Build history of the part. All positions in model axes, mm. A direction names the side the tool comes from. Round coordinates to 2 decimals unless told otherwise and drop trailing zeros. Loops run counter-clockwise (first coordinate to the right, second up) from the corner with the lowest first, then second, coordinate; pieces in that order, holes last. Notation, with made-up numbers: (31, 58.25) - (72, 58.25) arc R24 cw to (72, 73.25) - close; hole circle Ø11 at (-33.5, 32). An arc over 180 degrees is marked (long way). Use a Markdown table: item, result.
Autodesk Inventor part; units mm, degrees
ref_plane "РабПлоскость1" through (0, 0, 3) normal (0, 0, 1) x (1, 0, 0)
ref_plane "YZ Plane" through (0, 0, 0) normal (1, 0, 0) x (0, 1, 0)
ref_plane "XZ Plane" through (0, 0, 0) normal (0, 1, 0) x (-1, 0, 0)
ref_plane "РабПлоскость1" through (0, 0, 3) normal (0, 0, 1) x (1, 0, 0)
sketch "Эскиз1" plane through (0, 0, 3) normal (0, 0, 1) x (1, 0, 0)
  circle A0 centre (0, 0) radius 135
  circle A1 centre (0, 0) radius 101 construction
  line L0 (0, 0) -> (0, 184.3698) construction
  circle A2 centre (-37.8353, 93.6456) radius 27
  circle A3 centre (-92.2681, 41.0804) radius 27
  circle A4 centre (37.8353, 93.6456) radius 27
  circle A5 centre (92.2681, 41.0804) radius 27
  line L1 (0, 0) -> (37.8353, 93.6456) construction
  line L2 (0, 0) -> (92.2681, 41.0804) construction
  circle A6 centre (0, 0) radius 67
  line L3 (-135, 0) -> (135, 0)
  circle A7 centre (120, 0) radius 1.6 construction
  circle A8 centre (-120, 0) radius 1.6 construction
  circle A9 centre (120, 0) radius 8 construction
  circle A10 centre (-120, 0) radius 8 construction
  circle A11 centre (0, 120) radius 1.6 construction
  circle A12 centre (0, 120) radius 8 construction
  line L4 (0, 0) -> (-116.9134, -67.5) construction
  line L5 (0, 0) -> (116.9134, -67.5) construction
  point P0 (67, 0)
  point P1 (-67, 0)
  point P2 (-128, 0)
  point P3 (-112, 0)
  point P4 (112, 0)
  point P5 (128, 0)
  dimension "d0" = 54
  dimension "d3" = 202
  dimension "d4" = 34
  dimension "d5" = 34
  dimension "d9" = 16
  dimension "d11" = 120
  dimension "d12" = 22
  dimension "d13" = 44
extrude "Выдавливание1" add sketch "Эскиз1" along normal blind 6 contours L3 A6 A0 picked at (99.1742, 4.7591)
fillet "Сопряжение1" radius 5 4 edges at (-67, 0, 6) (-135, 0, 6) (67, 0, 6) (135, 0, 6)
equation "\"d5\" = d4"
equation "\"d13\" = 2 * d12"
properties part number "Фиксатор" material "По умолчанию1"
Q1. Drop flat-ended pins along their axis: pin 1 (2 mm diameter, centred on x = 14.5, z = 5, fed in from +Y); pin 2 (2 mm diameter, centred on x = 74.5, z = 6.5, fed in from +Y). Give the stop position or say it passes through.
Results found:
| item | result |
|---|---|
| pin 1 | stops at y = 134.32 |
| pin 2 | stops at y = 113.24 |
Q2. Cut at B-B, the plane x = -56.5. List the corners of the cut face in (y, z).
Results found:
| item | result |
|---|---|
| outline | (36.01, 3) - (74.14, 3) - (74.14, 9) - (36.01, 9) - close; (113.16, 3) - (122.61, 3) - (122.61, 9) - (113.16, 9) - close |
Q3. Which spindle directions (+Z, -Z, +X, -X, +Y, -Y) get a long thin tool onto all of the face, cutting with end or side? Do faces 4 (the face through (-68.45, 1.31, 6.04)), 5 (the face through (-66.515, 32.97, 5.958)). Say none if no direction does.
Results found:
| item | result |
|---|---|
| face 4 | +Z, -Z, -Y |
| face 5 | +Z, -Z |
Q4. Cut at C-C, the plane y = 117. List the corners of the cut face in (x, z).
Results found:
| item | result |
|---|---|
| outline | (-67.35, 3) - (-51.38, 3) - (-51.38, 9) - (-67.35, 9) - close; (-24.29, 3) - (24.29, 3) - (24.29, 9) - (-24.29, 9) - close; (51.38, 3) - (67.35, 3) - (67.35, 9) - (51.38, 9) - close |
Q5. Probe line 1 (X direction, y = 38, z = 4.2); line 2 (X direction, y = 76, z = 7.1); line 3 (X direction, y = 56, z = 4.3). List the from-to ranges inside material, lowest first.
Results found:
| item | result |
|---|---|
| line 1 | x = -129.54 to -119.09, -65.44 to -55.18, 55.18 to 65.44, 119.09 to 129.54 |
| line 2 | x = -111.58 to -58.27, -17.4 to 17.4, 58.27 to 111.58 |
| line 3 | x = -122.84 to -114.77, -69.76 to -36.78, 36.78 to 69.76, 114.77 to 122.84 |
Q6. Pull direction X, two halves, no side cores. Call faces 1 (the face through (133.467, 1.493, 6.042)), 2 (the face through (68.38, 1.38, 6.04)), 3 (the face through (-133.546, 1.574, 6.042)): pulls with the +X half, pulls with the -X half, needs draft (parallel to the pull), parting line crosses it, or undercut.
Results found:
| item | result |
|---|---|
| face 1 | pulls with the +X half |
| face 2 | undercut |
| face 3 | pulls with the -X half |
Q7. Cut at D-D, the plane z = 5.5. List the corners of the cut face in (x, y), plus the area to 3 significant figures.
Results found:
| item | result |
|---|---|
| outline | (-134.9, 5.19) arc R5 ccw to (-129.9, 0) - (-71.83, 0) arc R5 ccw to (-66.84, 4.65) arc R67 cw to (66.84, 4.65) arc R5 ccw to (71.83, 0) - (129.9, 0) arc R5 ccw to (134.9, 5.19) arc R135 ccw to start; hole circle Ø54 at (-92.27, 41.08); hole circle Ø54 at (-37.84, 93.65); hole circle Ø54 at (37.84, 93.65); hole circle Ø54 at (92.27, 41.08) |
| area | 12,400 mm2 |
Q8. Cut at A-A, the plane y = 38. List the corners of the cut face in (x, z), plus the area to 3 significant figures.
Results found:
| item | result |
|---|---|
| outline | (-129.54, 3) - (-119.09, 3) - (-119.09, 9) - (-129.54, 9) - close; (-65.44, 3) - (-55.18, 3) - (-55.18, 9) - (-65.44, 9) - close; (55.18, 3) - (65.44, 3) - (65.44, 9) - (55.18, 9) - close; (119.09, 3) - (129.54, 3) - (129.54, 9) - (119.09, 9) - close |
| area | 249 mm2 |
